Could you check a few things on this model? Use its own coordinates, in mm. Face numbers are marked on the shaded views. Coordinates: 2 decimals unless noted, no trailing zeros. Loops run counter-clockwise (first coordinate to the right, second up) from the corner with the lowest first, then second, coordinate; pieces in that order, holes last.
from build123d import *

# Parameters (mm, degrees)
F0_W          = 90
F0_H          = 18
F1_DEPTH      = 4
F1_DEPTH_BACK = 4
F2_SIZE       = 2.5
F4_D          = 6.5
F5_D          = 8.8
F7_D          = 4.5


with BuildPart() as f1:
    # F0 (on Front) → F1 (new body, two sides)
    with BuildSketch(Plane.XZ) as f1_sk:
        Rectangle(F0_W, F0_H)
    extrude(amount=F1_DEPTH)
    extrude(f1_sk.sketch, amount=-F1_DEPTH_BACK)

    # F2
    f2_edges = [f1.edges().sort_by_distance(p)[0] for p in [
        (-45, 0, -9),
        (45, 0, -9),
    ]]
    chamfer(f2_edges, length=F2_SIZE)

    # F4 (through all)
    with Locations(Plane.XZ.offset(4)):
        with Locations((-29, 0), (29, 0)):
            Hole(F4_D / 2)

    # F5 (through all)
    with Locations(Plane.XZ.offset(4)):
        with Locations((0, 0)):
            Hole(F5_D / 2)

    # F7 (through all)
    with Locations(Plane.XY.offset(9)):
        with Locations((-36, 0), (-12, 0), (12, 0), (36, 0)):
            Hole(F7_D / 2)


solid = f1.part
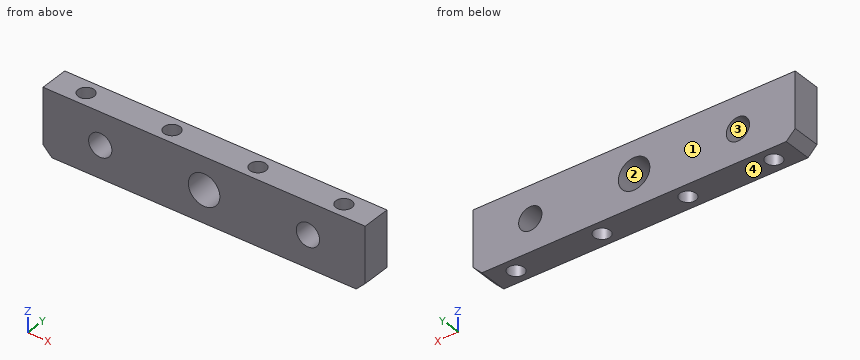
1) Imagine slicing it at D-D on z = 7.75. List the corners of the cut face in (x, y) for me, plus the area to 3 significant figures.
2) If I drill on L1, parallel to Y at x = -36, z = 1.5; L2, parallel to X at y = 0.75, z = -3.75; L3, parallel to Z at x = 0, y = 0.75, over which ranges is the centre line in solid material (lowest first)?
3) Imagine slicing it at C-C on y = -1. List the corners of the cut face in (x, z) for me, plus the area to 3 significant figures.
4) We'd pull the mould along Z, two halves only. Please class the marked faces 1, 2, 3 and 4: released by +Z, released by -Z, zero draft, split by the parting line, or undercut.
5) Imagine slicing it at B-B on x = 29. List the corners of the cut face in (y, z) for me.
6) Imagine slicing it at A-A on z = 0. List the corners of the cut face in (x, y) for me, plus the area to 3 significant figures.
Solved:
1. outline: (-45, -4) - (45, -4) - (45, 4) - (-45, 4) - close; hole circle Ø4.5 at (-36, 0); hole circle Ø4.5 at (-12, 0); hole circle Ø4.5 at (12, 0); hole circle Ø4.5 at (36, 0)
1. area: 656 mm2
2. L1: y = -4 to -2.25, 2.25 to 4
2. L2: x = -45 to -38.12, -33.88 to -14.12, -9.88 to -2.3, 2.3 to 9.88, 14.12 to 33.88, 38.12 to 45
2. L3: z = -9 to -4.4, 4.4 to 9
3. outline: (-45, -6.5) - (-42.5, -9) - (-38.02, -9) - (-38.02, 9) - (-45, 9) - close; (-33.98, -9) - (-14.02, -9) - (-14.02, 9) - (-33.98, 9) - close; (-9.98, -9) - (9.98, -9) - (9.98, 9) - (-9.98, 9) - close; (14.02, -9) - (33.98, -9) - (33.98, 9) - (14.02, 9) - close; (38.02, -9) - (42.5, -9) - (45, -6.5) - (45, 9) - (38.02, 9) - close; hole circle Ø6.5 at (-29, 0); hole circle Ø8.8 at (0, 0); hole circle Ø6.5 at (29, 0)
3. area: 1,200 mm2
4. face 1: zero draft
4. face 2: undercut
4. face 3: undercut
4. face 4: released by -Z
5. outline: (-4, -9) - (4, -9) - (4, -3.25) - (-4, -3.25) - close; (-4, 3.25) - (4, 3.25) - (4, 9) - (-4, 9) - close
6. outline: (-45, -4) - (-32.25, -4) - (-32.25, 4) - (-45, 4) - close; (-25.75, -4) - (-4.4, -4) - (-4.4, 4) - (-25.75, 4) - close; (4.4, -4) - (25.75, -4) - (25.75, 4) - (4.4, 4) - close; (32.25, -4) - (45, -4) - (45, 4) - (32.25, 4) - close; hole circle Ø4.5 at (-36, 0); hole circle Ø4.5 at (-12, 0); hole circle Ø4.5 at (12, 0); hole circle Ø4.5 at (36, 0)
6. area: 482 mm2
